Model file for the job. Use its own axes, mm. Face numbers are marked on the shaded views. A direction names the side the tool comes from. Coordinates: 2 decimals unless noted, no trailing zeros. Write each loop counter-clockwise with the first axis right and the second up, starting at its lowest first coordinate (ties: lowest second). Pieces come first, ordered by that corner, then holes. Notation, with made-up numbers: (57, 66) - (73, 66) arc R15 ccw to (73, 87) - close; hole circle Ø8 at (-30.75, -39). An arc over 180 degrees is marked (long way). Put each result on its own line as item: value. Start each with the question number.
1. Saw through at B-B, the plane y = -12. Write the cut outline in (x, z), plus the area to 3 significant figures.
2. Drop flat-ended pins along their axis: P1, Ø2.5, axis at y = -9.5, z = 1.5, coming from the -X side; P2, Ø0.5, axis at x = -2, z = 3.5, coming from the +Y side; P3, Ø1.3, axis at x = -15, y = -13, coming from the -Z side. Give the stop position or say it passes through.
3. Drill centre lines: L1, parallel to X at y = -10.25, z = 2.8; L2, parallel to Z at x = -7, y = -25; L3, parallel to Y at x = 15.5, z = 5.8. Where is each one in solid material? Low to high. Write a range as from..to.
4. Saw through at A-A, the plane z = 4.25. Write the cut outline in (x, y).
5. Which spindle directions (+Z, -Z, +X, -X, +Y, -Y) get a long thin tool onto all of the face, cutting with end or side? Do the marked faces 5, 6 and 7. Say none if no direction does.
6. Saw through at C-C, the plane z = 0.95. Write the cut outline in (x, y), plus the area to 3 significant figures.
7. Saw through at D-D, the plane x = 2.5. Write the cut outline in (y, z), plus the area to 3 significant figures.
8. Pull direction X, two halves, no side cores. Call the marked faces 1, 2, 3 and 4: released by +X, released by -X, zero draft, split by the parting line, or undercut.
```python
from build123d import *

# Parameters (mm, degrees)
F1_DEPTH       = 28.5
F5_DEPTH       = 2.5
F6_D           = 2
F6_CBORE_D     = 3
F6_CBORE_DEPTH = 1
F7_DEPTH       = 4
F8_W           = 10.6
F8_H           = 5
F9_DEPTH       = 1.75
F3_W           = 6.4
F3_H           = 4.7
F10_DEPTH      = 1.5


# Not quite as in the source:
# - ends of sketch curves that miss each other by under 0.0002 mm in the source are joined


with BuildPart() as f1:
    # F0 (on Front) → F1 (new body)
    with BuildSketch(Plane.XZ):
        Polygon((13.75, 6), (-13.75, 6), (-13.75, 0), (-11.8, 0), (-11.8, 4.7), (11.8, 4.7), (11.8, 0), (13.75, 0), align=None)
    extrude(amount=F1_DEPTH)

    # F4 (on face) → F5 (join)
    with BuildSketch(Plane.XY.offset(6)):
        with BuildLine():
            Line((-13.75, -7.4999997169), (-18.25, -7.4999997169))
            Line((-18.25, -7.4999997169), (-18.25, -16.4999997169))
            ThreePointArc((-18.25, -16.4999997169), (-15.0680194847, -17.8180192015), (-13.75, -20.9999997169))
            Line((-13.75, -20.9999997169), (-13.75, -7.4999997169))
        make_face()
        with BuildLine():
            Line((18.25, -7.4999999106), (13.75, -7.4999999106))
            Line((13.75, -7.4999999106), (13.75, -21))
            ThreePointArc((13.75, -21), (15.0680194847, -17.8180192015), (18.25, -16.4999997169))
            Line((18.25, -16.4999997169), (18.25, -7.4999999106))
        make_face()
    extrude(amount=-F5_DEPTH)

    # F6 (through all)
    with Locations(Plane.XY.offset(6)):
        with Locations((-16.05, -11.9999998212), (16.05, -11.9999998212)):
            CounterBoreHole(F6_D / 2, F6_CBORE_D / 2, F6_CBORE_DEPTH)

    # F3 (on face) → F7 (cut)
    with BuildSketch(Plane(origin=(0, 0, 0), x_dir=(-1, 0, 0), z_dir=(0, 1, 0))):
        Polygon((-5.4, 4.7), (-5.4, 0), (0, 0), (5.4, 0), (5.4, 4.7), (5.4, 6), (-5.4, 6), align=None)
    extrude(amount=-F7_DEPTH, mode=Mode.SUBTRACT)

    # F8 (on face) → F9 (join)
    with BuildSketch(Plane(origin=(0, 0, 4.7), x_dir=(1, 0, 0), z_dir=(0, 0, -1))):
        with Locations((0, 26)):
            Rectangle(F8_W, F8_H)
    extrude(amount=F9_DEPTH)

    # F3 (on face) → F10 (join)
    with BuildSketch(Plane(origin=(0, 0, 0), x_dir=(-1, 0, 0), z_dir=(0, 1, 0))):
        with Locations((-8.6, 2.35)):
            Rectangle(F3_W, F3_H)
        with Locations((8.6, 2.35)):
            Rectangle(F3_W, F3_H)
    extrude(amount=-F10_DEPTH)


solid = f1.part
```
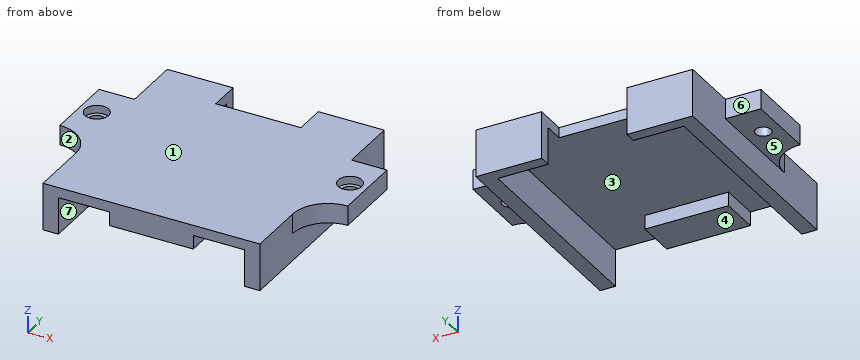
Final values:
1. outline: (-18.25, 3.5) - (-17.05, 3.5) - (-17.05, 5) - (-17.55, 5) - (-17.55, 6) - (-18.25, 6) - close; (-15.05, 3.5) - (-13.75, 3.5) - (-13.75, 0) - (-11.8, 0) - (-11.8, 4.7) - (11.8, 4.7) - (11.8, 0) - (13.75, 0) - (13.75, 3.5) - (15.05, 3.5) - (15.05, 5) - (14.55, 5) - (14.55, 6) - (-14.55, 6) - (-14.55, 5) - (-15.05, 5) - close; (17.05, 3.5) - (18.25, 3.5) - (18.25, 6) - (17.55, 6) - (17.55, 5) - (17.05, 5) - close
1. area: 64.6 mm²
2. P1: stops at x = -13.75
2. P2: stops at y = -23.5
2. P3: stops at z = 3.5
3. L1: x = -13.75..-11.8, 11.8..13.75
3. L2: z = 4.7..6
3. L3: y = -17.44..-13.4, -10.6..-7.5
4. outline: (-18.25, -16.5) arc R4.5 cw to (-13.75, -21) - (-13.75, -28.5) - (-11.8, -28.5) - (-11.8, -1.5) - (-5.4, -1.5) - (-5.4, 0) - (-13.75, 0) - (-13.75, -7.5) - (-18.25, -7.5) - close; (-5.3, -28.5) - (5.3, -28.5) - (5.3, -23.5) - (-5.3, -23.5) - close; (5.4, -1.5) - (11.8, -1.5) - (11.8, -28.5) - (13.75, -28.5) - (13.75, -21) arc R4.5 cw to (18.25, -16.5) - (18.25, -7.5) - (13.75, -7.5) - (13.75, 0) - (5.4, 0) - close; hole circle Ø2 at (-16.05, -12); hole circle Ø2 at (16.05, -12)
5. face 5: -Z, -X, +Y, -Y
5. face 6: +Z, -Z, -X, +Y
5. face 7: -Z, -Y
6. outline: (-13.75, -28.5) - (-11.8, -28.5) - (-11.8, -1.5) - (-5.4, -1.5) - (-5.4, 0) - (-13.75, 0) - close; (5.4, -1.5) - (11.8, -1.5) - (11.8, -28.5) - (13.75, -28.5) - (13.75, 0) - (5.4, 0) - close
6. area: 130 mm²
7. outline: (-28.5, 2.95) - (-23.5, 2.95) - (-23.5, 4.7) - (-4, 4.7) - (-4, 6) - (-28.5, 6) - close
7. area: 40.6 mm²
8. face 1: zero draft
8. face 2: released by -X
8. face 3: undercut
8. face 4: undercut
